Can you work these out from the model? Positions are in its coordinate system, mm. Face numbers are marked on the shaded views. Give positions to 0.01 mm unless a question says otherwise; leave off trailing zeros. Write each loop counter-clockwise with the first axis right and the second up, starting at its lowest first coordinate (ties: lowest second). Pieces come first, ordered by that corner, then holes.
1. Suppose I cut it at D-D (x = -19.5). Please give me the cut outline in (y, z).
2. Thinking about a two-plate mould opening in X: for the marked faces 1, 2, 3 and 4, which applies, pulls with the +X half, pulls with the -X half, needs draft (parallel to the pull), parting line crosses it, or undercut?
3. Suppose I cut it at C-C (z = 1). Give the number of separate pieces and of enclosed holes in the cut face, and give its area (3 significant figures).
4. If I drill on probe 1 along Y at (x, z) = (-34, 3); probe 2 along X at (y, z) = (-10.5, 7.5), over which ranges is the centre line in solid material (lowest first)?
5. I'm going to push flat-ended pins straight in: pin 1 (3 mm diameter, centred on x = 24.5, y = 17.5, fed in from +Z); pin 2 (4 mm diameter, centred on x = -5.5, y = 7, fed in from +Z). Where does each tip first touch, or does it pass through?
6. Suppose I cut it at A-A (x = 2.5). Please give me the cut outline in (y, z).
```python
from build123d import *

# Parameters (mm, degrees)
F0_W     = 24.66
F0_H     = 24.66
F0_W_2   = 24.68
F0_H_2   = 24.68
F1_DEPTH = 8
F2_DEPTH = 1
F3_R     = 7.99999


# Not quite as in the source:
# - a fillet or chamfer is up to 0.001 mm smaller than in the source, because OpenCascade refuses the exact size


with BuildPart() as f1:
    # F0 (on Top) → F1 (new body)
    with BuildSketch(Plane.XY):
        Polygon((-40, -40), (40, -40), (40, 40), (-40, 40), (-40, -13.34), align=None)
        with Locations((-26.67, -26.67)):
            Rectangle(F0_W, F0_H, mode=Mode.SUBTRACT)
        with Locations((0, -26.67)):
            Rectangle(F0_W_2, F0_H, mode=Mode.SUBTRACT)
        with Locations((26.67, -26.67)):
            Rectangle(F0_W, F0_H, mode=Mode.SUBTRACT)
        with Locations((-26.67, 0)):
            Rectangle(F0_W, F0_H_2, mode=Mode.SUBTRACT)
        with Locations((-26.67, 26.67)):
            Rectangle(F0_W, F0_H, mode=Mode.SUBTRACT)
        Rectangle(F0_W_2, F0_H_2, mode=Mode.SUBTRACT)
        with Locations((26.67, 0)):
            Rectangle(F0_W, F0_H_2, mode=Mode.SUBTRACT)
        with Locations((0, 26.67)):
            Rectangle(F0_W_2, F0_H, mode=Mode.SUBTRACT)
        with Locations((26.67, 26.67)):
            Rectangle(F0_W, F0_H, mode=Mode.SUBTRACT)
    extrude(amount=F1_DEPTH)

    # F0 (on Top) → F2 (join)
    with BuildSketch(Plane.XY):
        Polygon((-40, -40), (40, -40), (40, 40), (-40, 40), (-40, -13.34), align=None)
        with Locations((-26.67, -26.67)):
            Rectangle(F0_W, F0_H, mode=Mode.SUBTRACT)
        with Locations((0, -26.67)):
            Rectangle(F0_W_2, F0_H, mode=Mode.SUBTRACT)
        with Locations((26.67, -26.67)):
            Rectangle(F0_W, F0_H, mode=Mode.SUBTRACT)
        with Locations((-26.67, 0)):
            Rectangle(F0_W, F0_H_2, mode=Mode.SUBTRACT)
        with Locations((-26.67, 26.67)):
            Rectangle(F0_W, F0_H, mode=Mode.SUBTRACT)
        Rectangle(F0_W_2, F0_H_2, mode=Mode.SUBTRACT)
        with Locations((26.67, 0)):
            Rectangle(F0_W, F0_H_2, mode=Mode.SUBTRACT)
        with Locations((0, 26.67)):
            Rectangle(F0_W_2, F0_H, mode=Mode.SUBTRACT)
        with Locations((26.67, 26.67)):
            Rectangle(F0_W, F0_H, mode=Mode.SUBTRACT)
        Rectangle(F0_W_2, F0_H_2)
        with Locations((-26.67, 0)):
            Rectangle(F0_W, F0_H_2)
        with Locations((0, -26.67)):
            Rectangle(F0_W_2, F0_H)
        with Locations((26.67, 0)):
            Rectangle(F0_W, F0_H_2)
        with Locations((0, 26.67)):
            Rectangle(F0_W_2, F0_H)
        with Locations((-26.67, -26.67)):
            Rectangle(F0_W, F0_H)
        with Locations((-26.67, 26.67)):
            Rectangle(F0_W, F0_H)
        with Locations((26.67, -26.67)):
            Rectangle(F0_W, F0_H)
        with Locations((26.67, 26.67)):
            Rectangle(F0_W, F0_H)
    extrude(amount=-F2_DEPTH)

    # F3 (radius 8 in the source; OpenCascade refuses exactly that, so slightly less here)
    f3_edges = [f1.edges().sort_by_distance(p)[0] for p in [
        (14.34, -26.67, 0),
        (14.34, 0, 0),
        (14.34, 26.67, 0),
        (-12.34, 26.67, 0),
        (-12.34, 0, 0),
        (-12.34, -26.67, 0),
        (-39, -26.67, 0),
        (-39, 0, 0),
        (-39, 26.67, 0),
        (12.34, -26.67, 0),
        (12.34, 0, 0),
        (12.34, 26.67, 0),
        (-14.34, 26.67, 0),
        (-14.34, 0, 0),
        (-14.34, -26.67, 0),
        (39, 26.67, 0),
        (39, 0, 0),
        (39, -26.67, 0),
    ]]
    fillet(f3_edges, radius=F3_R)


solid = f1.part
```
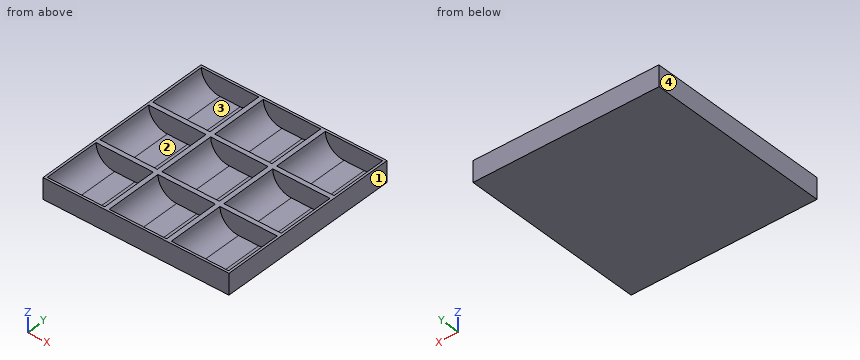
Checks:
1. outline: (-40, -1) - (40, -1) - (40, 8) - (39, 8) - (39, 0.52) - (14.34, 0.52) - (14.34, 8) - (12.34, 8) - (12.34, 0.52) - (-12.34, 0.52) - (-12.34, 8) - (-14.34, 8) - (-14.34, 0.52) - (-39, 0.52) - (-39, 8) - (-40, 8) - close
2. face 1: pulls with the +X half
2. face 2: undercut
2. face 3: undercut
2. face 4: pulls with the -X half
3. separate pieces: 1
3. enclosed holes: 9
3. area: 2,760 mm2
4. probe 1: y = -40 to -39, -14.34 to -12.34, 12.34 to 14.34, 39 to 40
4. probe 2: x = -40 to -38.98, -14.36 to -12.32, 12.32 to 14.36, 38.98 to 40
5. pin 1: stops at z = 0
5. pin 2: stops at z = 0.65
6. outline: (-40, -1) - (40, -1) - (40, 8) - (39, 8) - (39, 0) - (14.34, 0) - (14.34, 8) - (12.34, 8) - (12.34, 0) - (-12.34, 0) - (-12.34, 8) - (-14.34, 8) - (-14.34, 0) - (-39, 0) - (-39, 8) - (-40, 8) - close
